Geometry check sheet. Reference: the model listing, model coordinates, mm. A direction names the side the tool comes from. Coordinates: 2 decimals unless noted, no trailing zeros. Write each loop counter-clockwise with the first axis right and the second up, starting at its lowest first coordinate (ties: lowest second). Pieces come first, ordered by that corner, then holes. Notation, with made-up numbers: (43, 39.25) -> (64, 39.25) arc R19 cw to (64, 56.25) -> close; hole circle Ø10 at (-12, 37.5). An arc over 180 degrees is marked (long way). Answer in a Markdown table with one row per item. Add a question column.
Q1. Gauge pin test, flat ends, axial feed: P1, Ø1.3, axis at x = -78.5, z = 2, coming from the +Y side; P2, Ø1.3, axis at x = -72, z = 1.5, coming from the -Y side. Record the tip position at first contact, or that the pin passes through.
Q2. Tool access check on faces 1 (the face through (-79.1, 10, 2)), 2 (the face through (61, 15, 2)), 3 (the face through (-75, 5, 2)), 4 (the face through (-61, 15, 2)). Record the directions out of +Z, -Z, +X, -X, +Y, -Y that give a thin tool (end or side, any length) a straight path to the whole face; none if there is none.
Q3. Section check A-A, the plane x = 61.5. Record the boundary of the cut face in (y, z), and give its area (3 significant figures).
Q4. Release check for a two-part mould opening along Y. For faces 5 (the face through (75, -15, 2)), 6 (the face through (-1, 0, 0)), 7 (the face through (79.1, 10, 2)) record: pulls with the +Y half, pulls with the -Y half, needs draft (parallel to the pull), parting line crosses it, or undercut.
Q5. Thickness scan on line 1 (X direction, y = 10.5, z = 2.9); line 2 (X direction, y = 7.5, z = 3.05); line 3 (Y direction, x = 55, z = 1.75). Record the ranges inside material, lowest first.
```python
from build123d import *

# Parameters (mm, degrees)
SKETCH1_W           = 200
SKETCH1_H           = 30
SKETCH1_W_2         = 100
SKETCH1_H_2         = 6
BOSS_EXTRUDE1_DEPTH = 4
SKETCH2_W           = 5
SKETCH2_H           = 20
SKETCH2_W_2         = 8.2
SKETCH2_H_2         = 4
CUT_EXTRUDE1_DEPTH  = 10


with BuildPart() as part:
    # Sketch1 → Boss-Extrude1 (new body)
    with BuildSketch(Plane.XY):
        Rectangle(SKETCH1_W, SKETCH1_H)
        with Locations((0, -15)):
            Rectangle(SKETCH1_W_2, SKETCH1_H_2)
        with Locations((0, 15)):
            Rectangle(SKETCH1_W_2, SKETCH1_H_2)
    extrude(amount=BOSS_EXTRUDE1_DEPTH)

    # Sketch2 → Cut-Extrude1 (cut)
    with BuildSketch(Plane.XY.offset(4)):
        with Locations((-75, 15)):
            Rectangle(SKETCH2_W, SKETCH2_H)
        with Locations((-75, 10)):
            Rectangle(SKETCH2_W_2, SKETCH2_H_2)
    cut_extrude1 = extrude(amount=-CUT_EXTRUDE1_DEPTH, mode=Mode.SUBTRACT)

    # Mirror1: Cut-Extrude1 across plane
    add(cut_extrude1.mirror(Plane(origin=(0, 0, 0), x_dir=(0, 0, 1), z_dir=(1, 0, 0))), mode=Mode.SUBTRACT)


solid = part.part
```
Calculated:
| question | item | result |
|---|---|---|
| 1 | P1 | stops at y = 15 |
| 1 | P2 | stops at y = -15 |
| 2 | face 1 | +Z, -Z |
| 2 | face 2 | +Z, -Z, +X, +Y |
| 2 | face 3 | +Z, -Z, +Y |
| 2 | face 4 | +Z, -Z, -X, +Y |
| 3 | outline | (-15, 0) -> (15, 0) -> (15, 4) -> (-15, 4) -> close |
| 3 | area | 120 mm² |
| 4 | face 5 | pulls with the -Y half |
| 4 | face 6 | needs draft |
| 4 | face 7 | undercut |
| 5 | line 1 | x = -100 to -79.1, -70.9 to 70.9, 79.1 to 100 |
| 5 | line 2 | x = -100 to -77.5, -72.5 to 72.5, 77.5 to 100 |
| 5 | line 3 | y = -15 to 15 |
